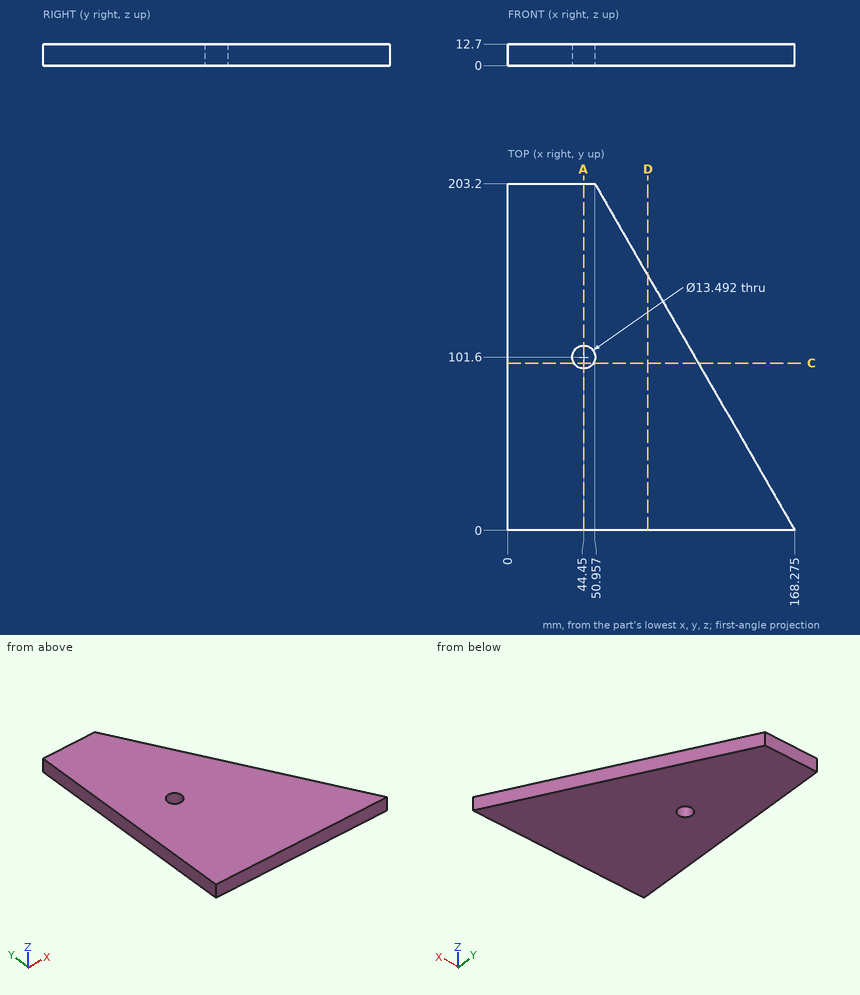
Check sheet for the drawn part. Datum: minimum x, y, z corner. Units: mm. Give positions to 0.01 mm unless a question says otherwise; leave off trailing zeros. Write each loop counter-clockwise with the first axis right and the second up, starting at its lowest first coordinate (ties: lowest second). Pieces come first, ordered by that corner, then holes.
(1) Cross-section at A-A (x = 44.45). Enter the section's corners in (y, z).
(2) Cross-section at D-D (x = 82). Enter the section's corners in (y, z), plus the area to 3 significant figures.
(3) Cross-section at C-C (y = 98). Enter the section's corners in (x, z) (1 decimal).
(4) Gauge pin test, flat ends, axial feed: pin 1 (2 mm diameter, centred on y = 167.5, z = 2, fed in from +X) (1 decimal); pin 2 (5 mm diameter, centred on y = 90, z = 3, fed in from +X). Record the tip position at first contact, or that the pin passes through.
(5) Material ranges on line 1 (Y direction, x = 44.45, z = 8); line 2 (Y direction, x = 143, z = 6.5) (1 decimal); line 3 (X direction, y = 136, z = 8) (1 decimal), recorded low to high.
Worked out:
1. outline: (0, 0) - (94.85, 0) - (94.85, 12.7) - (0, 12.7) - close; (108.35, 0) - (203.2, 0) - (203.2, 12.7) - (108.35, 12.7) - close
2. outline: (0, 0) - (149.43, 0) - (149.43, 12.7) - (0, 12.7) - close
2. area: 1,900 mm2
3. outline: (0, 0) - (38.7, 0) - (38.7, 12.7) - (0, 12.7) - close; (50.2, 0) - (111.7, 0) - (111.7, 12.7) - (50.2, 12.7) - close
4. pin 1: stops at x = 72.1
4. pin 2: stops at x = 117.76
5. line 1: y = 0 to 94.85, 108.35 to 203.2
5. line 2: y = 0 to 43.8
5. line 3: x = 0 to 89.8
